For this review, take the finished solid that the model builds, in its own axes (mm). A direction names the side the tool comes from. Coordinates: 2 decimals unless noted, no trailing zeros. Loops run counter-clockwise (first coordinate to the right, second up) from the corner with the lowest first, then second, coordinate; pieces in that order, holes last. Notation, with made-up numbers: (88, -6.5) - (147, -6.5) arc R25 cw to (147, 22.5) - close; hole circle Ø5 at (83.5, 29). An arc over 180 degrees is marked (long way). Answer as a JSON object with one key per item and string values. Group by question number.
Item 1: We need section B-B (z = -29). Give the boundary of the cut face in (x, y), then the cut area to 3 significant figures.
Item 2: We need section C-C (z = -69.5). Give the boundary of the cut face in (x, y), then the cut area to 3 significant figures.
Item 3: Tool access review of faces 1 (the conical face through (-0.16, 1.222, -40.56)), 2 (the flat face through (0, 0, 0)): name each direction out of +Z, -Z, +X, -X, +Y, -Y from which nothing blocks a thin tool from reaching the whole face with its end or side.
Item 4: Clearance check with flat-ended pins moving along their axes: pin 1 (2.5 mm diameter, centred on x = 0, z = -2, fed in from -Y); pin 2 (2.5 mm diameter, centred on x = 0, z = -2, fed in from +Y); pin 3 (1.5 mm diameter, centred on x = -2, y = 1.5, fed in from +Z). State where each tip first meets the part, or that it passes through.
Item 5: To check wall thickness, follow line 1 (X direction, y = 0.6, z = -2); line 2 (X direction, y = 1.45, z = -2); line 3 (X direction, y = 0.3, z = -28). State the ranges of each line that lie inside material, in increasing order.
from build123d import *

# Parameters (mm, degrees)
SKETCH4_R               = 1.5
CUT_EXTRUDE3_DEPTH      = 3.5
CUT_EXTRUDE3_DEPTH_BACK = 3.5
SKETCH7_R               = 1
CUT_EXTRUDE4_DEPTH      = 3.5000001
CUT_EXTRUDE4_DEPTH_BACK = 3.5000001


with BuildPart() as part:
    # Sketch2 → Revolve2 (revolve)
    with BuildSketch(Plane(origin=(0, 0, 0), x_dir=(1, 0, 0), z_dir=(0, 1, 0))):
        Polygon((0, 0), (2.5, 0), (0, 80), align=None)
    revolve(axis=Axis((0, 0, -80), (0, 0, 1)))

    # Sketch4 → Cut-Extrude3 (cut, two sides)
    with BuildSketch(Plane(origin=(0, 0, 0), x_dir=(1, 0, 0), z_dir=(0, 1, 0))) as cut_extrude3_sk:
        with Locations((0, 15)):
            Circle(SKETCH4_R)
    extrude(amount=CUT_EXTRUDE3_DEPTH, mode=Mode.SUBTRACT)
    extrude(cut_extrude3_sk.sketch, amount=-CUT_EXTRUDE3_DEPTH_BACK, mode=Mode.SUBTRACT)

    # Sketch7 → Cut-Extrude4 (cut, two sides)
    with BuildSketch(Plane(origin=(0, 0, 0), x_dir=(1, 0, 0), z_dir=(0, 1, 0))) as cut_extrude4_sk:
        with Locations((0, 2)):
            Circle(SKETCH7_R)
    extrude(amount=CUT_EXTRUDE4_DEPTH, mode=Mode.SUBTRACT)
    extrude(cut_extrude4_sk.sketch, amount=-CUT_EXTRUDE4_DEPTH_BACK, mode=Mode.SUBTRACT)


solid = part.part
Check sheet entries:
{
 "1": {"outline": "circle Ø3.19 at (0, 0)", "area": "7.98 mm2"},
 "2": {"outline": "circle Ø0.66 at (0, 0)", "area": "0.338 mm2"},
 "3": {"face 1": "-Z", "face 2": "+Z, +X, -X, +Y, -Y"},
 "4": {"pin 1": "stops at y = -2.48", "pin 2": "stops at y = 2.48", "pin 3": "stops at z = 0"},
 "5": {"line 1": "x = -2.36 to -1, 1 to 2.36", "line 2": "x = -1.96 to -1, 1 to 1.96", "line 3": "x = -1.6 to 1.6"}
}
